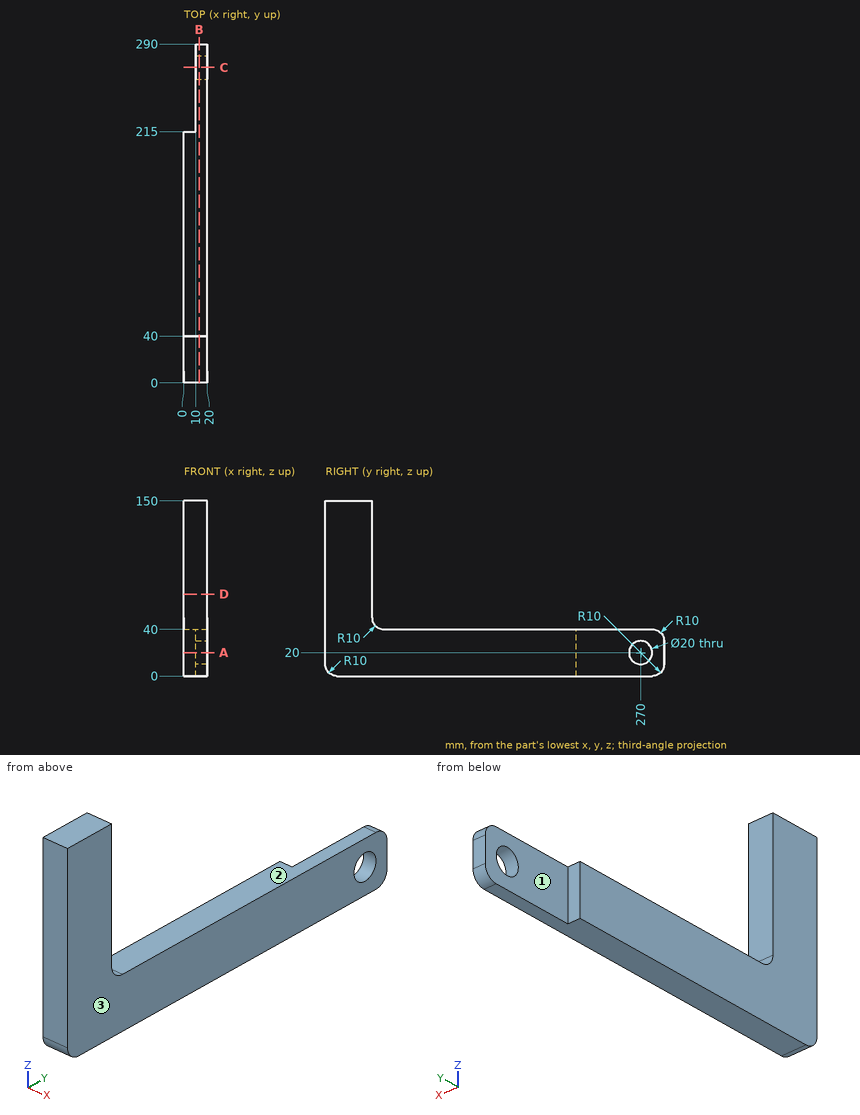
Job drawing, mm, ordinate dimensions from the low corner. One solid piece. A direction names the side the tool comes from. Give positions to 0.01 mm unless a question says otherwise; leave off trailing zeros. Loops run counter-clockwise (first coordinate to the right, second up) from the corner with the lowest first, then second, coordinate; pieces in that order, holes last. Notation, with made-up numbers: M 1,59.5 L 29,59.5 A34 cw 29,91.5 Z; hole C 48,31.5 d5. An arc over 180 degrees is marked long. Answer in a Markdown table with one row per item. Add a question column.
Item 1: Band-saw the part on A-A on z = 20. Give the cut face in (x, y).
Item 2: Probe probe 1 along Z at (x, y) = (16, 270); probe 2 along Y at (x, z) = (13.25, 20); probe 3 along Z at (x, y) = (12.5, 80). List the from-to ranges inside material, lowest first.
Item 3: Drop flat-ended pins along their axis: P1, Ø1.5, axis at x = 16, y = 224.5, coming from the +Z side; P2, Ø10, axis at x = 14, z = 112, coming from the +Y side. Give the stop position or say it passes through.
Item 4: Tool access for the marked faces 1, 2 and 3: list every direction of +Z, -Z, +X, -X, +Y, -Y with a clear straight run to the whole face (end or side of a thin tool).
Item 5: Band-saw the part on D-D on z = 70. Give the cut face in (x, y).
Item 6: Band-saw the part on C-C on y = 270. Give the cut face in (x, z).
Item 7: Band-saw the part on B-B on x = 13. Give the cut face in (y, z), then the cut area to 3 significant figures.
Reply:
| question | item | result |
|---|---|---|
| 1 | outline | M 0,0 L 20,0 L 20,260 L 10,260 L 10,215 L 0,215 Z; M 10,280 L 20,280 L 20,290 L 10,290 Z |
| 2 | probe 1 | z = 0 to 10, 30 to 40 |
| 2 | probe 2 | y = 0 to 260, 280 to 290 |
| 2 | probe 3 | z = 0 to 40 |
| 3 | P1 | stops at z = 40 |
| 3 | P2 | stops at y = 40 |
| 4 | face 1 | +Z, -Z, -X, +Y |
| 4 | face 2 | +Z, +X, -X, +Y |
| 4 | face 3 | +Z, -Z, +X, +Y, -Y |
| 5 | outline | M 0,0 L 20,0 L 20,40 L 0,40 Z |
| 6 | outline | M 10,0 L 20,0 L 20,10 L 10,10 Z; M 10,30 L 20,30 L 20,40 L 10,40 Z |
| 7 | outline | M 0,10 A10 ccw 10,0 L 280,0 A10 ccw 290,10 L 290,30 A10 ccw 280,40 L 50,40 A10 cw 40,50 L 40,150 L 0,150 Z; hole C 270,20 d20 |
| 7 | area | 15,600 mm^2 |
